Geometry check sheet. Reference: the model listing, model coordinates, mm. A direction names the side the tool comes from. Coordinates: 2 decimals unless noted, no trailing zeros. Loops run counter-clockwise (first coordinate to the right, second up) from the corner with the lowest first, then second, coordinate; pieces in that order, holes last. Notation, with made-up numbers: (-38.5, 63.5) - (-18.5, 63.5) arc R29 ccw to (-18.5, 95.5) - close; hole circle Ø1 at (7.25, 7). An arc over 180 degrees is marked (long way). Write each question's results on one line, items separated by ' | '. Start each with the question number.
(1) Sectioned sample at C-C (z = 5.5). State how many separate pieces and enclosed holes the cut face has, plus the area to 3 significant figures.
(2) Access from +Z, -Z, +X, -X, +Y, -Y to the whole of each face (thin tool, end or side, straight path). Record for faces 4 (the face through (21.755, -39, 4)), 5 (the face through (26.976, -19, 4)).
(3) Sectioned sample at B-B (x = 5.5). Enter the section's corners in (y, z).
(4) Sectioned sample at D-D (y = -40). Enter the section's corners in (x, z).
(5) Material ranges on probe 1 along X at (y, z) = (9, 1.25); probe 2 along Y at (x, z) = (22.5, 7.25); probe 3 along X at (y, z) = (-2, 2.25), recorded low to high.
(6) Mould release check, pull along Y, two halves, no side actions. Record for faces 1 (the face through (-26.554, 29.668, 3.698)), 2 (the face through (0.707, 9, 4)), 3 (the face through (-22.89, 42.02, 3.7)): pulls with the +Y half, pulls with the -Y half, needs draft (parallel to the pull), parting line crosses it, or undercut.
(7) Go/stop test with flat-tipped pins: pin 1 Ø2 at (y, z) = (-2.5, 5.5) entering from -X; pin 2 Ø2 at (y, z) = (-40.5, 4.5) entering from +X; pin 3 Ø10 at (x, y) = (-17.5, -1.5) entering from +Z; pin 4 Ø2 at (x, z) = (-6, 6.5) entering from +Y. Record where each tip stops, or that it passes through.
(8) Sectioned sample at A-A (y = -11.5). Enter the section's corners in (x, z), plus the area to 3 significant figures.
from build123d import *

# Parameters (mm, degrees)
SKETCH_1_R      = 8.137429072
EXTRUDE_1_DEPTH = 7.5


with BuildPart() as part:
    # 草图1 → 凸台-拉伸1 (new body)
    with BuildSketch(Plane.XY):
        Polygon((10.655742112, -51.13350276), (26.975655976, -51.132648268), (26.975655976, -45.355975578), (24.381633836, -45.338595321), (21.754811222, -46.744598553), (21.754811222, -31.335745249), (24.341110056, -32.847488843), (26.975655976, -32.865266967), (26.975655976, -3.94984418), (24.423395969, -3.952666276), (21.754811222, -5.399476315), (21.754811222, 10.078826219), (24.3888497, 8.498393016), (26.975655976, 8.501001852), (26.975655976, 14.3375467), (26.975655976, 33.668056688), (9.607760849, 47.75359746), (-4.011253891, 51.18832036), (-18.902979431, 48.177822313), (-26.990082321, 35.687740526), (-26.106294212, 23.478023729), (-20.096405563, 13.353512011), (-10.914003906, 4.339931688), (-1.275932846, -17.697925367), (2.140880051, -26.591846266), align=None)
        with Locations((-5.684087388, 32.581137097)):
            Circle(SKETCH_1_R, mode=Mode.SUBTRACT)
        Polygon((0.706809044, 7.273735046), (0.706809044, 11.775535583), (11.016924858, 18.016654968), (11.016924858, -18.659224532), align=None, mode=Mode.SUBTRACT)
    extrude(amount=EXTRUDE_1_DEPTH)


solid = part.part
Outcome:
1) separate pieces: 1 | enclosed holes: 2 | area: 2,990 mm2
2) face 4: +Z, -Z | face 5: +Z, -Z, +X, +Y, -Y
3) outline: (-36.27, 0) - (-4.78, 0) - (-4.78, 7.5) - (-36.27, 7.5) - close; (14.68, 0) - (48.79, 0) - (48.79, 7.5) - (14.68, 7.5) - close
4) outline: (6.79, 0) - (21.75, 0) - (21.75, 7.5) - (6.79, 7.5) - close
5) probe 1: x = -15.66 to 0.71, 11.02 to 21.75, 23.55 to 26.98 | probe 2: y = -51.13 to -46.35, -31.77 to -5, 9.63 to 37.3 | probe 3: x = -8.14 to 4.39, 11.02 to 21.75
6) face 1: pulls with the -Y half | face 2: undercut | face 3: pulls with the +Y half
7) pin 1: stops at x = -8.36 | pin 2: stops at x = 21.75 | pin 3: passes through | pin 4: stops at y = 50.99
8) outline: (-3.99, 0) - (8.17, 0) - (8.17, 7.5) - (-3.99, 7.5) - close; (11.02, 0) - (26.98, 0) - (26.98, 7.5) - (11.02, 7.5) - close | area: 211 mm2
